from build123d import *

# Parameters (mm, degrees)
SKETCH1_R           = 11
BOSS_EXTRUDE1_DEPTH = 3
SKETCH2_R           = 1.5
CUT_EXTRUDE1_DEPTH  = 3
SKETCH3_R           = 3.5
SKETCH3_R_2         = 2
BOSS_EXTRUDE2_DEPTH = 2


with BuildPart() as part:
    # Sketch1 → Boss-Extrude1 (new body)
    with BuildSketch(Plane.XY):
        Circle(SKETCH1_R)
    extrude(amount=BOSS_EXTRUDE1_DEPTH)

    # Sketch2 → Cut-Extrude1 (cut)
    with BuildSketch(Plane.XY.offset(3)):
        with Locations((0, 8)):
            Circle(SKETCH2_R)
        with Locations((-8, 0)):
            Circle(SKETCH2_R)
        with Locations(Location((0, -8, 0), (0, 0, 180))):
            Circle(SKETCH2_R)
        with Locations(Location((8, 0, 0), (0, 0, 180))):
            Circle(SKETCH2_R)
    extrude(amount=-CUT_EXTRUDE1_DEPTH, mode=Mode.SUBTRACT)

    # Sketch3 → Boss-Extrude2 (add)
    with BuildSketch(Plane.XY.offset(3)):
        Circle(SKETCH3_R)
        Circle(SKETCH3_R_2, mode=Mode.SUBTRACT)
    extrude(amount=BOSS_EXTRUDE2_DEPTH)


solid = part.part
Geometry check sheet. Reference: the model listing, model coordinates, mm. A direction names the side the tool comes from. Give positions to 0.01 mm unless a question says otherwise; leave off trailing zeros. Order: outer loops, then holes, each group sorted by start corner. A loop starts at its lowest first (then second) coordinate and runs counter-clockwise, first axis right, second up.
1. Depth check by flat-ended pin: pin 1 (1.5 mm diameter, centred on x = 6.5, z = 1, fed in from -Y); pin 2 (3.5 mm diameter, centred on x = 0, y = 0, fed in from +Z); pin 3 (1 mm diameter, centred on x = -7, z = 4, fed in from +Y); pin 4 (1 mm diameter, centred on y = -4, z = 2, fed in from -X). Enter the tip coordinate at first touch or a pass-through.
Completed:
pin 1: stops at y = -9.38
pin 2: stops at z = 3
pin 3: passes through
pin 4: stops at x = -10.43
2. Access from +Z, -Z, +X, -X, +Y, -Y to the whole of each face (thin tool, end or side, straight path). Record for faces 4 (the face through (-9.5, 0.07, 1.52)), 5 (the face through (3.233, -1.341, 3.986)).
Completed:
face 4: +Z, -Z
face 5: +Z
3. Sectioned sample at C-C (y = -8). Record the boundary of the cut face in (x, z), then the cut area to 3 significant figures.
Completed:
outline: (-7.55, 0) - (-1.5, 0) - (-1.5, 3) - (-7.55, 3) - close; (1.5, 0) - (7.55, 0) - (7.55, 3) - (1.5, 3) - close
area: 36.3 mm2
4. Draft check along Y on faces 1 (the face through (0, 0, 0)), 2 (the face through (-2.38, -10.74, 1.48)), 3 (the face through (0, 0, 3)). Enter one of: pulls with the +Y half, pulls with the -Y half, needs draft (parallel to the pull), parting line crosses it, or undercut.
Completed:
face 1: needs draft
face 2: parting line crosses it
face 3: undercut
5. Sectioned sample at A-A (y = 0.5). Record the boundary of the cut face in (x, z), then the cut area to 3 significant figures.
Completed:
outline: (-10.99, 0) - (-9.41, 0) - (-9.41, 3) - (-10.99, 3) - close; (-6.59, 0) - (6.59, 0) - (6.59, 3) - (3.46, 3) - (3.46, 5) - (1.94, 5) - (1.94, 3) - (-1.94, 3) - (-1.94, 5) - (-3.46, 5) - (-3.46, 3) - (-6.59, 3) - close; (9.41, 0) - (10.99, 0) - (10.99, 3) - (9.41, 3) - close
area: 55.1 mm2
6. Sectioned sample at B-B (z = 1.55). Record the boundary of the cut face in (x, y).
Completed:
outline: circle Ø22 at (0, 0); hole circle Ø3 at (-8, 0); hole circle Ø3 at (0, -8); hole circle Ø3 at (0, 8); hole circle Ø3 at (8, 0)
7. Scan lines: line 1 (Y direction, x = 0, z = 1.45); line 2 (X direction, y = 0.75, z = 1.7); line 3 (Z direction, x = 9.25, y = 1.5). Record each from-to range of solid material in increasing order.
Completed:
line 1: y = -11 to -9.5, -6.5 to 6.5, 9.5 to 11
line 2: x = -10.97 to -9.3, -6.7 to 6.7, 9.3 to 10.97
line 3: z = 0 to 3
